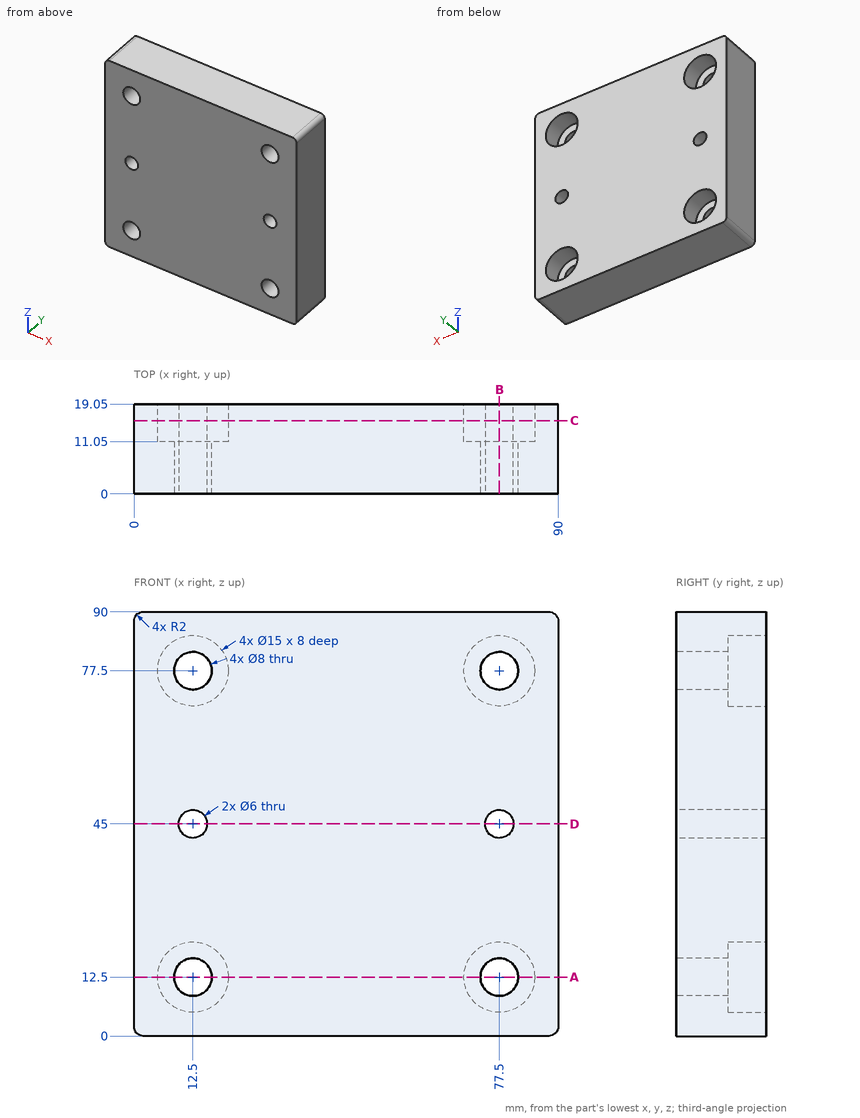
Input: dimensioned drawing with shaded views. Units: mm. Origin: part minimum x, y, z. Round coordinates to 2 decimals unless told otherwise and drop trailing zeros. Order: outer loops, then holes, each group sorted by start corner. A loop starts at its lowest first (then second) coordinate and runs counter-clockwise, first axis right, second up. Notation, with made-up numbers: (89, -15.75) - (121, -15.75) arc R12 cw to (121, 0.25) - close; hole circle Ø6 at (13.25, 62.25). An arc over 180 degrees is marked (long way). Write item = value, one per line. Start each with the question number.
Q1. Cut plane D-D on z = 45. Return the cut outline in (x, y), and give its area (3 significant figures).
Q2. Cut plane B-B on x = 77.5. Return the cut outline in (y, z).
Q3. Cut plane C-C on y = 15.5. Return the cut outline in (x, z).
Q4. Cut plane A-A on z = 12.5. Return the cut outline in (x, y), and give its area (3 significant figures).
Q5. Pin query (flat end, axial travel): pin 1 (5.5 mm diameter, centred on x = 77.5, z = 45, fed in from +Y); pin 2 (10.5 mm diameter, centred on x = 12.5, z = 12.5, fed in from +Y). Return the tip coordinate at first contact, or that it passes through.
Q6. Ray query, line 1 (X direction, y = 4, z = 12.5); line 2 (Z direction, x = 12.5, y = 17); line 3 (X direction, y = 13.75, z = 12.5). Return the intervals inside material, ascending. Write a range as from..to.
Outcome:
q1.outline = (0, 0) - (9.5, 0) - (9.5, 19.05) - (0, 19.05) - close; (15.5, 0) - (74.5, 0) - (74.5, 19.05) - (15.5, 19.05) - close; (80.5, 0) - (90, 0) - (90, 19.05) - (80.5, 19.05) - close
q1.area = 1,490 mm^2
q2.outline = (0, 0) - (19.05, 0) - (19.05, 5) - (11.05, 5) - (11.05, 8.5) - (0, 8.5) - close; (0, 16.5) - (11.05, 16.5) - (11.05, 20) - (19.05, 20) - (19.05, 42) - (0, 42) - close; (0, 48) - (19.05, 48) - (19.05, 70) - (11.05, 70) - (11.05, 73.5) - (0, 73.5) - close; (0, 81.5) - (11.05, 81.5) - (11.05, 85) - (19.05, 85) - (19.05, 90) - (0, 90) - close
q3.outline = (0, 2) arc R2 ccw to (2, 0) - (88, 0) arc R2 ccw to (90, 2) - (90, 88) arc R2 ccw to (88, 90) - (2, 90) arc R2 ccw to (0, 88) - close; hole circle Ø15 at (12.5, 12.5); hole circle Ø15 at (12.5, 77.5); hole circle Ø6 at (12.5, 45); hole circle Ø15 at (77.5, 12.5); hole circle Ø15 at (77.5, 77.5); hole circle Ø6 at (77.5, 45)
q4.outline = (0, 0) - (8.5, 0) - (8.5, 11.05) - (5, 11.05) - (5, 19.05) - (0, 19.05) - close; (16.5, 0) - (73.5, 0) - (73.5, 11.05) - (70, 11.05) - (70, 19.05) - (20, 19.05) - (20, 11.05) - (16.5, 11.05) - close; (81.5, 0) - (90, 0) - (90, 19.05) - (85, 19.05) - (85, 11.05) - (81.5, 11.05) - close
q4.area = 1,300 mm^2
q5.pin_1 = through
q5.pin_2 = 11.05
q6.line_1 = 0..8.5, 16.5..73.5, 81.5..90
q6.line_2 = 0..5, 20..42, 48..70, 85..90
q6.line_3 = 0..5, 20..70, 85..90
